Here's the drawing with two shaded views (mm, measured from the low corner). I have some questions. Give positions to 0.01 mm unless a question says otherwise; leave off trailing zeros. Loops run counter-clockwise (first coordinate to the right, second up) from the corner with the lowest first, then second, coordinate; pieces in that order, holes last. Notation, with made-up numbers: (-16.5, 33.5) - (33.5, 33.5) arc R21 ccw to (33.5, 71.5) - close; hole circle Ø4 at (-6.5, -27). An arc over 180 degrees is marked (long way). Use one line per item in the form item = value.
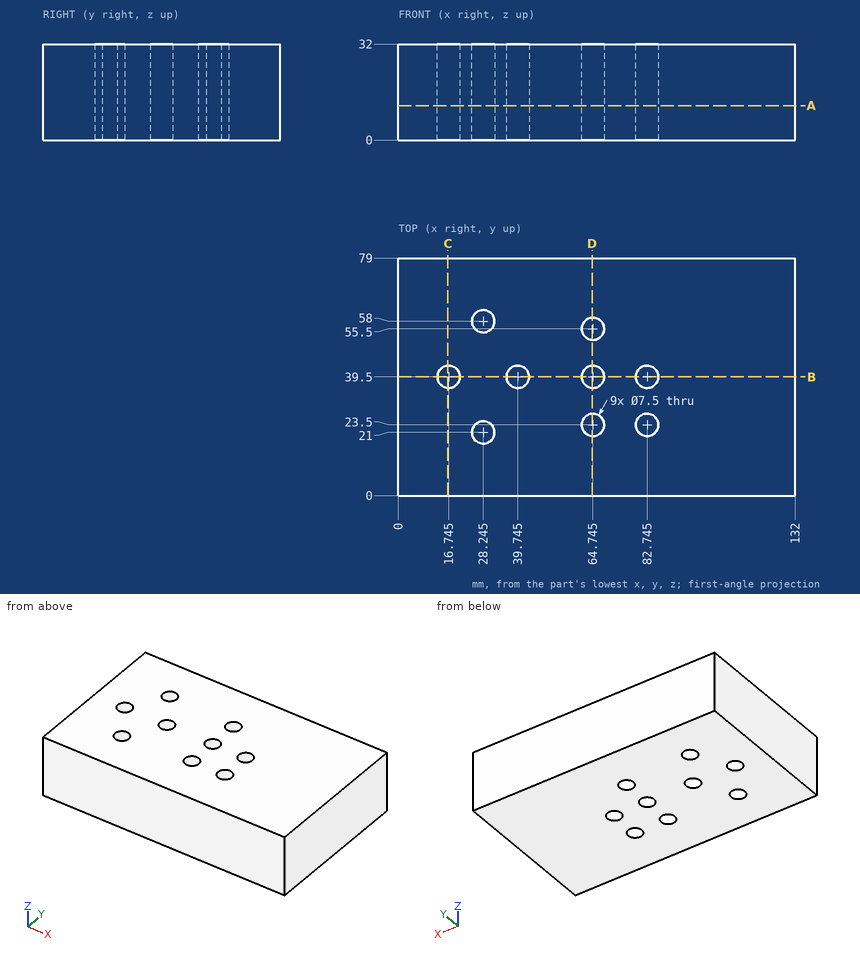
(1) For P1, Ø7, axis at x = 28.24, y = 21, coming from the +Z side, with a flat end and sliding along its axis, tell me the tip position at first contact or that it passes through.
Geometry says:
P1 = through
(2) If I drill on probe 1 along X at (y, z) = (23, 14); probe 2 along X at (y, z) = (39, 22); probe 3 along X at (y, z) = (41.5, 19.5), over which ranges is the centre line in solid material (lowest first)?
Geometry says:
probe_1 = 0 to 25.07, 31.42 to 61.03, 68.46 to 79.03, 86.46 to 132
probe_2 = 0 to 13.03, 20.46 to 36.03, 43.46 to 61.03, 68.46 to 79.03, 86.46 to 132
probe_3 = 0 to 13.57, 19.92 to 36.57, 42.92 to 61.57, 67.92 to 79.57, 85.92 to 132
(3) If we section it at B-B (y = 39.5): List the corners of the cut face in (x, z) for me (3 decimals), plus the area to 3 significant figures.
Geometry says:
outline = (0, 0) - (12.995, 0) - (12.995, 32) - (0, 32) - close; (20.495, 0) - (35.995, 0) - (35.995, 32) - (20.495, 32) - close; (43.495, 0) - (60.995, 0) - (60.995, 32) - (43.495, 32) - close; (68.495, 0) - (78.995, 0) - (78.995, 32) - (68.495, 32) - close; (86.495, 0) - (132, 0) - (132, 32) - (86.495, 32) - close
area = 3,260 mm²
(4) If we section it at A-A (z = 11.5): Give the number of separate pieces and of enclosed holes in the cut face, plus the area to 3 significant figures.
Geometry says:
separate_pieces = 1
enclosed_holes = 9
area = 10,000 mm²
(5) If we section it at D-D (x = 64.5): List the corners of the cut face in (y, z) for me.
Geometry says:
outline = (0, 0) - (19.76, 0) - (19.76, 32) - (0, 32) - close; (27.24, 0) - (35.76, 0) - (35.76, 32) - (27.24, 32) - close; (43.24, 0) - (51.76, 0) - (51.76, 32) - (43.24, 32) - close; (59.24, 0) - (79, 0) - (79, 32) - (59.24, 32) - close
(6) If we section it at C-C (x = 16.5): List the corners of the cut face in (y, z) for me.
Geometry says:
outline = (0, 0) - (35.76, 0) - (35.76, 32) - (0, 32) - close; (43.24, 0) - (79, 0) - (79, 32) - (43.24, 32) - close
